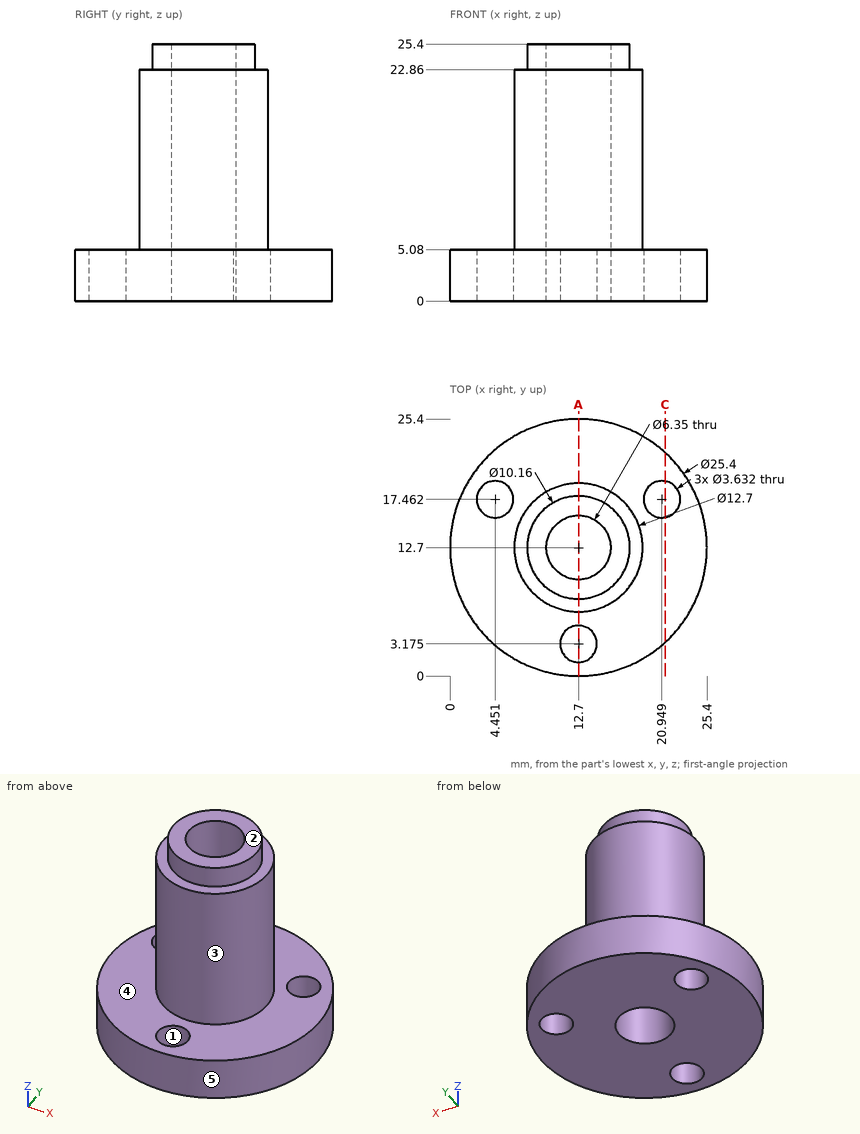
Part print with two shaded views. Sizes in mm from the minimum x, y, z corner. A direction names the side the tool comes from. Round coordinates to 2 decimals unless told otherwise and drop trailing zeros. Order: outer loops, then holes, each group sorted by start corner. A loop starts at its lowest first (then second) coordinate and runs counter-clockwise, first axis right, second up.
(1) 3-axis set-ups, long thin cutter, end or side, ignore diameter. For the marked faces 4 and 5: which of +Z, -Z, +X, -X, +Y, -Y reach the whole face in a straight line?
(2) Band-saw the part on C-C (x = 21.25). List the corners of the cut face in (y, z).
(3) Drill centre lines: line 1 (Z direction, x = 12.75, y = 20); line 2 (Z direction, x = 7.75, y = 10.5); line 3 (Y direction, x = 13.25, z = 20.5) (1 decimal). Where is each one in solid material? Low to high.
(4) Pull direction X, two halves, no side cores. Call the marked faces 1, 2 and 3: released by +X, released by -X, zero draft, split by the parting line, or undercut.
(5) Pin check, flat tips, straight feed: pin 1 (5 mm diameter, centred on y = 7.5, z = 5, fed in from -X); pin 2 (2 mm diameter, centred on x = 7, z = 8, fed in from +Y); pin 3 (5 mm diameter, centred on y = 7, z = 15, fed in from -X) (1 decimal). Stop position of each tip, or through.
(6) Band-saw the part on A-A (x = 12.7). Give the number of separate pieces and of enclosed holes in the cut face, then the cut area to 3 significant figures.
Verdict:
1. face 4: +Z
1. face 5: +Z, -Z
2. outline: (3.31, 0) - (15.67, 0) - (15.67, 5.08) - (3.31, 5.08) - close; (19.25, 0) - (22.09, 0) - (22.09, 5.08) - (19.25, 5.08) - close
3. line 1: z = 0 to 5.08
3. line 2: z = 0 to 22.86
3. line 3: y = 6.4 to 9.6, 15.8 to 19
4. face 1: undercut
4. face 2: zero draft
4. face 3: split by the parting line
5. pin 1: stops at x = 0.29
5. pin 2: stops at y = 16.97
5. pin 3: stops at x = 7.2
6. separate pieces: 3
6. enclosed holes: 0
6. area: 201 mm2
